```python
from build123d import *

# Parameters (mm, degrees)
SKETCH1_W           = 100.584
SKETCH1_H           = 53.34
SKETCH1_R           = 3.302
BOSS_EXTRUDE2_DEPTH = 5.08
SKETCH5_W           = 60.96
SKETCH5_H           = 53.34
BOSS_EXTRUDE3_DEPTH = 19.05
CUT_EXTRUDE4_REACH  = 55.34
SKETCH6_R           = 25.4
SKETCH7_W           = 100.584
SKETCH7_H           = 26.67
CUT_EXTRUDE5_DEPTH  = 25.13


with BuildPart() as part:
    # Sketch1 → Boss-Extrude2 (new body)
    with BuildSketch(Plane.XY):
        with Locations((-9.978006062, 1.929359203)):
            Rectangle(SKETCH1_W, SKETCH1_H)
        with Locations((30.661993938, 20.725359203)):
            Circle(SKETCH1_R, mode=Mode.SUBTRACT)
        with Locations((30.661993938, -16.866640797)):
            Circle(SKETCH1_R, mode=Mode.SUBTRACT)
        with Locations((-50.618006062, 20.725359203)):
            Circle(SKETCH1_R, mode=Mode.SUBTRACT)
        with Locations((-50.618006062, -16.866640797)):
            Circle(SKETCH1_R, mode=Mode.SUBTRACT)
    extrude(amount=BOSS_EXTRUDE2_DEPTH)

    # Sketch5 → Boss-Extrude3 (add)
    with BuildSketch(Plane.XY.offset(5.08)):
        with Locations((-9.978006062, 1.929359203)):
            Rectangle(SKETCH5_W, SKETCH5_H)
    extrude(amount=BOSS_EXTRUDE3_DEPTH)

    # Sketch6 → Cut-Extrude4 (cut, up to next)
    with BuildSketch(Plane.XZ.offset(24.740640797), mode=Mode.PRIVATE) as cut_extrude4_sk1:
        with Locations((-9.978006062, 30.48)):
            Circle(SKETCH6_R)
    cut_extrude4_tool1 = extrude(cut_extrude4_sk1.sketch, amount=-CUT_EXTRUDE4_REACH, mode=Mode.PRIVATE) & part.part
    add(cut_extrude4_tool1.solids().sort_by_distance((-9.978006, -24.740641, 30.48))[0], mode=Mode.SUBTRACT)

    # Sketch7 → Cut-Extrude5 (cut, through all)
    with BuildSketch(Plane(origin=(0, 0, 0), x_dir=(-1, 0, 0), z_dir=(0, 0, -1))):
        with Locations((9.978006062, -11.405640797)):
            Rectangle(SKETCH7_W, SKETCH7_H)
    extrude(amount=-CUT_EXTRUDE5_DEPTH, mode=Mode.SUBTRACT)


solid = part.part
```
Model file for the job. Use its own axes, mm. A direction names the side the tool comes from. Coordinates: 2 decimals unless noted, no trailing zeros. Loops run counter-clockwise (first coordinate to the right, second up) from the corner with the lowest first, then second, coordinate; pieces in that order, holes last. Notation, with made-up numbers: (56, 62.5) - (114, 62.5) arc R22 cw to (114, 84.5) - close; hole circle Ø6 at (72.5, -17). An arc over 180 degrees is marked (long way). Answer as a JSON object with one key per item and string values. Group by question number.
(1) Probe line 1 along X through (y, z) = (18.5, 2.75); line 2 along X through (y, z) = (7.5, 8); line 3 along Z through (x, y) = (-9, 11.25). List the from-to ranges inside material, lowest first.
(2) Flat gauge pins, fed straight in: pin 1 (5 mm diameter, centred on x = -8.5, y = 23.5, fed in from +Z); pin 2 (2 mm diameter, centred on y = 18.5, z = 21, fed in from +X); pin 3 (16 mm diameter, centred on x = -54.5, y = 10.5, fed in from +Z). Where does each tip first touch, or does it go through?
(3) Tool access for faces 4 (the face through (30, 15, 5.08)), 5 (the face through (40.314, 15, 3)), 6 (the face through (-40.458, 15, 14)): list every direction of +Z, -Z, +X, -X, +Y, -Y with a clear straight run to the whole face (end or side of a thin tool).
(4) Cut at B-B (y = 22.25). Give the cut face in (x, z).
(5) Cut at D-D (y = 5.75). Give the cut face in (x, z).
(6) Two-plate mould, pull along X, no slides. Class faces 1 (the face through (-53.917, 20.871, 2.504)), 2 (the face through (-51, 15, 5.08)), 3 (the face through (20.502, 15, 14)): released by +X, released by -X, zero draft, split by the parting line, or undercut.
(7) Cut at C-C (x = 33). Give the cut face in (y, z), then the cut area to 3 significant figures.
(8) Cut at A-A (z = 15.5). Give the cut face in (x, y).
Geometry says:
{
 "1": {"line 1": "x = -60.27 to -53.06, -48.18 to 28.22, 33.1 to 40.31", "line 2": "x = -40.46 to -21.8, 1.85 to 20.5", "line 3": "z = 0 to 5.1"},
 "2": {"pin 1": "stops at z = 5.39", "pin 2": "stops at x = 20.5", "pin 3": "stops at z = 5.08"},
 "3": {"face 4": "+Z, +X, +Y, -Y", "face 5": "+Z, -Z, +X, +Y, -Y", "face 6": "+Z, -X, +Y, -Y"},
 "4": {"outline": "(-60.27, 0) - (-53.55, 0) - (-53.55, 5.08) - (-60.27, 5.08) - close; (-47.69, 0) - (27.73, 0) - (27.73, 5.08) - (20.5, 5.08) - (20.5, 24.13) - (14.62, 24.13) arc R25.4 cw to (-34.57, 24.13) - (-40.46, 24.13) - (-40.46, 5.08) - (-47.69, 5.08) - close; (33.59, 0) - (40.31, 0) - (40.31, 5.08) - (33.59, 5.08) - close"},
 "5": {"outline": "(-60.27, 0) - (40.31, 0) - (40.31, 5.08) - (20.5, 5.08) - (20.5, 24.13) - (14.62, 24.13) arc R25.4 cw to (-34.57, 24.13) - (-40.46, 24.13) - (-40.46, 5.08) - (-60.27, 5.08) - close"},
 "6": {"face 1": "undercut", "face 2": "zero draft", "face 3": "released by +X"},
 "7": {"outline": "(1.93, 0) - (18.39, 0) - (18.39, 5.08) - (1.93, 5.08) - close; (23.06, 0) - (28.6, 0) - (28.6, 5.08) - (23.06, 5.08) - close", "area": "112 mm^2"},
 "8": {"outline": "(-40.46, 1.93) - (-30.49, 1.93) - (-30.49, 28.6) - (-40.46, 28.6) - close; (10.53, 1.93) - (20.5, 1.93) - (20.5, 28.6) - (10.53, 28.6) - close"}
}
